Read the model definition and answer for the solid it produces. Units are mm, in the model's axes. A direction names the side the tool comes from. Coordinates: 2 decimals unless noted, no trailing zeros. Write each loop counter-clockwise with the first axis right and the second up, starting at its lowest first coordinate (ties: lowest second). Pieces come first, ordered by that corner, then holes.
1) Find the intervals of material crossed by line 1 (Z direction, x = -31, y = -10); line 2 (Z direction, x = -62, y = -4.5); line 3 (Y direction, x = -26, z = 12), in increasing order.
2) Which of the six approach directions +Z, -Z, +X, -X, +Y, -Y give full straight-line access (tool end or side, diameter ignored) to faces 1 (the face through (-29.49, -15.62, -3.47)), 2 (the face through (-0.5, 4.72, 14.98))?
3) The part is cut by section A-A (x = -33.5). Determine the outline of the cut face in (y, z), then the cut area to 3 significant figures.
4) The part is cut by section B-B (x = -51.5). Determine the outline of the cut face in (y, z).
5) Each of these flat-tipped pins is pushed along its axis until it touches: pin 1 Ø4 at (x, z) = (-23, -2) entering from -Y; pin 2 Ø3 at (x, y) = (-27.5, 3) entering from -Z; pin 3 Ø2 at (x, y) = (-15.5, 20) entering from +Z. Where does it stop, or does it pass through?
from build123d import *


with BuildPart() as f1:
    # F0 (on Front) → F1 (revolve)
    with BuildSketch(Plane.XZ):
        with BuildLine():
            Line((0, 15.100086289), (-7.9947902337, 24.7891377658))
            add(Edge.make_bspline(
                [(-13.5336209388, 25.8130880211), (-13.1794829922, 26.0396653478), (-12.3469790571, 26.5077257402), (-10.9534140953, 26.5328921513), (-9.365299038, 26.0844114305), (-8.2402056984, 25.1083988869), (-8.0565123354, 24.8694320839), (-7.9947902337, 24.7891377658)],
                knots=[0.0753740232, 0.0753740232, 0.0753740232, 0.0753740232, 0.236653892, 0.4524170896, 0.6819552068, 0.89313499, 1, 1, 1, 1], degree=3))
            Line((-13.5336209388, 25.8130880211), (-19.239403379, 20.4293505417))
            ThreePointArc((-19.239403379, 20.4293505417), (-19.7032923995, 19.7667886958), (-19.8668379088, 18.9746813235))
            Line((-19.8668379088, 18.9746813235), (-19.8668367383, 17.0000005928))
            ThreePointArc((-19.8668367383, 17.0000005928), (-20.1597297475, 16.2928934284), (-20.8668367383, 16))
            Line((-20.8668367383, 16), (-37.8668361455, 16))
            ThreePointArc((-37.8668361455, 16), (-38.5739429267, 15.7071067812), (-38.8668361455, 15))
            Line((-38.8668361455, 15), (-38.8668361455, 13.5))
            ThreePointArc((-38.8668361455, 13.5), (-39.1597293643, 12.7928932188), (-39.8668361455, 12.5))
            Line((-39.8668361455, 12.5), (-65.8668361455, 12.5))
            Line((-65.8668361455, 12.5), (-65.8668361455, 0))
            Line((-65.8668361455, 0), (-26.8668361455, 0))
            Line((-26.8668361455, 0), (-19.8668361455, 0))
            Line((-19.8668361455, 0), (0, 0))
            Line((0, 0), (0, 15.100086289))
        make_face()
    revolve(axis=Axis((-46.3668361455, 0, 0), (-1, 0, 0)))


solid = f1.part
Reported:
1. line 1: z = -12.49 to 12.49
1. line 2: z = -11.66 to 11.66
1. line 3: y = -10.58 to 10.58
2. face 1: -X
2. face 2: +X
3. outline: circle Ø32 at (0, 0)
3. area: 804 mm2
4. outline: circle Ø25 at (0, 0)
5. pin 1: stops at y = -16
5. pin 2: stops at z = -15.93
5. pin 3: stops at z = 15.31
